```python
from build123d import *

# Parameters (mm, degrees)
SKETCH_1_R          = 17.5
SKETCH_1_R_2        = 5
EXTRUDE_1_DEPTH     = 16
SKETCH_2_R          = 8
SKETCH_2_R_2        = 5
EXTRUDE_2_DEPTH     = 2
SKETCH_3_R          = 3.5
CUT_EXTRUDE_1_DEPTH = 12


with BuildPart() as part:
    # 草图1 → 凸台-拉伸1 (new body)
    # profile 1 of 2: a face of its own
    with BuildSketch(Plane.XY):
        with BuildLine():
            Line((-33.5, 6), (-33.5, 0))
            Line((-33.5, 0), (33.5, 0))
            Line((33.5, 0), (33.5, 6))
            Line((33.5, 6), (21.332723466, 6))
            Line((21.332723466, 6), (16.90370196, 22.529333289))
            ThreePointArc((16.90370196, 22.529333289), (17.350285074, 20.284208364), (17.5, 18))
            ThreePointArc((17.5, 18), (-2.284208364, 0.649714926), (-16.90370196, 22.529333289))
            Line((-16.90370196, 22.529333289), (-21.332723466, 6))
            Line((-21.332723466, 6), (-33.5, 6))
        make_face()
    # profile 2 of 2: a face of its own
    with BuildSketch(Plane.XY):
        with Locations((0, 18)):
            Circle(SKETCH_1_R)
        with Locations((0, 18)):
            Circle(SKETCH_1_R_2, mode=Mode.SUBTRACT)
    extrude(amount=EXTRUDE_1_DEPTH)

    # 草图2 → 凸台-拉伸2 (add)
    with BuildSketch(Plane.XY.offset(16)):
        with Locations((0, 18)):
            Circle(SKETCH_2_R)
        with Locations((0, 18)):
            Circle(SKETCH_2_R_2, mode=Mode.SUBTRACT)
    extrude(amount=EXTRUDE_2_DEPTH)

    # 草图3 → 切除-拉伸1 (cut)
    with BuildSketch(Plane(origin=(0, 6, 0), x_dir=(1, 0, 0), z_dir=(0, 1, 0))):
        with Locations(Location((-26.5, -8, 0), (0, 0, 270))):
            Circle(SKETCH_3_R)
        with Locations(Location((26.5, -8, 0), (0, 0, 180))):
            Circle(SKETCH_3_R)
    extrude(amount=-CUT_EXTRUDE_1_DEPTH, mode=Mode.SUBTRACT)


solid = part.part
```
The model under review builds one solid part; all positions refer to its coordinate system, in mm. A direction names the side the tool comes from. Give positions to 0.01 mm unless a question says otherwise; leave off trailing zeros. Write each loop counter-clockwise with the first axis right and the second up, starting at its lowest first coordinate (ties: lowest second). Pieces come first, ordered by that corner, then holes.
(1) Consider section C-C, the plane z = 2.75. Give the boundary of the cut face in (x, y).
(2) The part is to be moulded in two halves that separate along X. For faces 1 (the flat face through (-0.1, 12.8, 18)), 2 (the cylindrical face through (-23, 3, 8)), 3 (the flat face through (19.15, 14.15, 7.89)), say which applies: released by +X, released by -X, zero draft, split by the parting line, or undercut.
(3) Tool access review of faces 4 (the flat face through (30.2, 6, 7.9)), 5 (the cylindrical face through (-1.08, 13.12, 8.87)), 6 (the cylindrical face through (-1.73, 10.19, 16.99)), 7 (the flat face through (-30, 6, 6)): name each direction out of +Z, -Z, +X, -X, +Y, -Y from which nothing blocks a thin tool from reaching the whole face with its end or side.
(4) Consider section D-D, the plane y = 18. Give the boundary of the cut face in (x, z).
(5) Consider section A-A, the plane z = 8. Give the boundary of the cut face in (x, y), and give its area (3 significant figures).
(6) To check wall thickness, follow L1, parallel to Z at x = -6, y = 7.5; L2, parallel to Y at x = -26, z = 13.5; L3, parallel to X at y = 16.5, z = 13.75. State the ranges of each line that lie inside material, in increasing order.
(7) Consider section B-B, the plane x = 26.5. Give the boundary of the cut face in (y, z).
(8) For P1, Ø6, axis at y = 20, z = 10.5, coming from the -X side; P2, Ø6, axis at x = 0, y = 18, coming from the -Z side; P3, Ø1, axis at x = 11, y = 26.5, coming from the -Z side; P4, Ø8, axis at x = 26.5, z = 8, coming from the +Y side, all flat-tipped, find the tip position at first contact; note any pin that passes through.
Returned:
1. outline: (-33.5, 0) - (33.5, 0) - (33.5, 6) - (21.33, 6) - (16.9, 22.53) arc R17.5 ccw to (-16.9, 22.53) - (-21.33, 6) - (-33.5, 6) - close; hole circle Ø10 at (0, 18)
2. face 1: zero draft
2. face 2: undercut
2. face 3: released by +X
3. face 4: +Z, -Z, +X, +Y
3. face 5: +Z, -Z
3. face 6: +Z
3. face 7: +Z, -Z, -X, +Y
4. outline: (-18.12, 0) - (-5, 0) - (-5, 18) - (-8, 18) - (-8, 16) - (-18.12, 16) - close; (5, 0) - (18.12, 0) - (18.12, 16) - (8, 16) - (8, 18) - (5, 18) - close
5. outline: (-33.5, 0) - (-30, 0) - (-30, 6) - (-33.5, 6) - close; (-23, 0) - (23, 0) - (23, 6) - (21.33, 6) - (16.9, 22.53) arc R17.5 ccw to (-16.9, 22.53) - (-21.33, 6) - (-23, 6) - close; (30, 0) - (33.5, 0) - (33.5, 6) - (30, 6) - close; hole circle Ø10 at (0, 18)
5. area: 1,200 mm2
6. L1: z = 0 to 16
6. L2: y = 0 to 6
6. L3: x = -18.52 to -4.77, 4.77 to 18.52
7. outline: (0, 0) - (6, 0) - (6, 4.5) - (0, 4.5) - close; (0, 11.5) - (6, 11.5) - (6, 16) - (0, 16) - close
8. P1: stops at x = -18.39
8. P2: passes through
8. P3: stops at z = 0
8. P4: stops at y = 6
